```python
from build123d import *

# Parameters (mm, degrees)
CUT_EXTRUDE3_DEPTH      = 141.1869469
CUT_EXTRUDE3_DEPTH_BACK = 141.1869469
SKETCH8_OUTSIDE_W       = 46.838
SKETCH8_OUTSIDE_H       = 46.838
SKETCH8_OUTSIDE_W_2     = 13.97
SKETCH8_OUTSIDE_H_2     = 13.97
CUT_EXTRUDE4_DEPTH      = 141.186946801


with BuildPart() as part:
    # Sketch1 → Revolve3 (revolve)
    with BuildSketch(Plane.XY, mode=Mode.PRIVATE) as revolve3_sk:
        with BuildLine():
            Line((0, 0), (0, 2.54))
            Line((0, 2.54), (82.55, 2.54))
            Line((82.55, 2.54), (82.55, 6.985))
            ThreePointArc((82.55, 6.985), (82.921974388, 7.883025612), (83.82, 8.255))
            Line((83.82, 8.255), (85.01103416, 8.255))
            ThreePointArc((85.01103416, 8.255), (85.64603416, 8.084852263), (86.110886423, 7.62))
            ThreePointArc((86.110886423, 7.62), (92.71, 3.81), (99.309113577, 7.62))
            ThreePointArc((99.309113577, 7.62), (99.77396584, 8.084852263), (100.40896584, 8.255))
            Line((100.40896584, 8.255), (133.35, 8.255))
            ThreePointArc((133.35, 8.255), (137.840128061, 6.395128061), (139.7, 1.905))
            Line((139.7, 1.905), (139.7, 0))
            Line((139.7, 0), (0, 0))
        make_face()
    revolve(revolve3_sk.sketch.rotate(Axis((-862.051792103, 0, 0), (1, 0, 0)), 90), axis=Axis((-862.051792103, 0, 0), (1, 0, 0)))

    # Sketch5 → Cut-Extrude3 (cut, two sides: drawn at the far end of the back side and taken through both)
    with BuildSketch(Plane.XY.offset(-CUT_EXTRUDE3_DEPTH_BACK)):
        Polygon((270.361206931, -33.513682078), (18.100809936, -2.54), (0, -0.3175), (0, 0.3175), (18.100809936, 2.54), (270.361206931, 33.513682078), (-237.948450162, 33.513682078), (-237.948450162, -33.513682078), align=None)
    extrude(amount=CUT_EXTRUDE3_DEPTH + CUT_EXTRUDE3_DEPTH_BACK, mode=Mode.SUBTRACT)

    # Sketch8 outside → Cut-Extrude4 (cut, through all)
    with BuildSketch(Plane(origin=(139.7, 0, 0), x_dir=(0, 0, -1), z_dir=(1, 0, 0))):
        Rectangle(SKETCH8_OUTSIDE_W, SKETCH8_OUTSIDE_H)
        Rectangle(SKETCH8_OUTSIDE_W_2, SKETCH8_OUTSIDE_H_2, mode=Mode.SUBTRACT)
    extrude(amount=-CUT_EXTRUDE4_DEPTH, mode=Mode.SUBTRACT)


solid = part.part
```
Design review of the part built by this model. Coordinates are the model's own, in mm. A direction names the side the tool comes from. Round coordinates to 2 decimals unless told otherwise and drop trailing zeros. Write each loop counter-clockwise with the first axis right and the second up, starting at its lowest first coordinate (ties: lowest second). Pieces come first, ordered by that corner, then holes.
Item 1: We need section A-A on x = 111. Write out the cut boundary in (y, z) (3 decimals).
Item 2: For probe 1 along X at (y, z) = (-1.25, 6); probe 2 along X at (y, z) = (-2.5, -3.75); probe 3 along Z at (x, y) = (60.5, 0.25), list the stretches that pass through material, from the lowest coordinate up.
Item 3: We need section B-B on x = 55. Write out the cut boundary in (y, z).
Item 4: For faces 5 (the flat face through (82.55, 0, -3)), 6 (the flat face through (6.912, 1.166, -0.035)), list the 3-axis set-ups (+Z, -Z, +X, -X, +Y, -Y) from which the entire face can be reached by the end or side of a thin tool; tool diameter is ignored.
Item 5: The part is to be moulded in two halves that separate along Z. For faces 1 (the flat face through (139.7, 0, 0)), 2 (the cylindrical face through (84.424, -5.855, -5.819)), 3 (the cylindrical face through (51.03, -1.72, -1.87)), 4 (the flat face through (118, 0, 6.985)), say which applies: +Z half, -Z half, draft (parallel to the pull), parting line (faces both ways), or undercut.
Item 6: Clearance check with flat-ended pins moving along their axes: pin 1 Ø4 at (y, z) = (-2, 3.5) entering from -X; pin 2 Ø4 at (x, y) = (18, -2.5) entering from -Z; pin 3 Ø3 at (x, z) = (46, -1.5) entering from -Y; pin 4 Ø1 at (x, z) = (21.5, 2.5) entering from +Y. State where each tip first meets the part, or that it passes through.
Returned:
1. outline: (-6.985, -4.399) arc R8.255 ccw to (-4.399, -6.985) - (4.399, -6.985) arc R8.255 ccw to (6.985, -4.399) - (6.985, 4.399) arc R8.255 ccw to (4.399, 6.985) - (-4.399, 6.985) arc R8.255 ccw to (-6.985, 4.399) - close
2. probe 1: x = 82.55 to 87.24, 98.18 to 138.09
2. probe 2: x = 82.55 to 89.53, 95.89 to 139.14
2. probe 3: z = -2.53 to 2.53
3. outline: circle Ø5.08 at (0, 0)
4. face 5: -X
4. face 6: +Z, -Z, -X, +Y
5. face 1: draft
5. face 2: -Z half
5. face 3: parting line
5. face 4: +Z half
6. pin 1: stops at x = 0
6. pin 2: stops at z = -2.49
6. pin 3: stops at y = -2.54
6. pin 4: stops at y = 1.57
